from build123d import *

# Parameters (mm, degrees)
SKETCH1_R           = 5.75
BOSS_EXTRUDE1_DEPTH = 1
SKETCH2_R           = 5
BOSS_EXTRUDE2_DEPTH = 3
SKETCH3_R           = 1.5
CUT_EXTRUDE1_DEPTH  = 10.06228448
SKETCH4_R           = 762
SKETCH4_R_2         = 4
CUT_EXTRUDE2_DEPTH  = 0.08
CUT_EXTRUDE3_START  = -0.08
SKETCH5_R           = 4
SKETCH5_R_2         = 2.5
CUT_EXTRUDE3_DEPTH  = 0.08
FILLET1_R           = 0.31


with BuildPart() as part:
    # Sketch1 → Boss-Extrude1 (new body)
    with BuildSketch(Plane(origin=(0, 0, 0), x_dir=(1, 0, 0), z_dir=(0, 1, 0))):
        with Locations(Location((0, 0, 0), (0, 0, 270))):
            Circle(SKETCH1_R)
    extrude(amount=BOSS_EXTRUDE1_DEPTH)

    # Sketch2 → Boss-Extrude2 (add)
    with BuildSketch(Plane(origin=(0, 1, 0), x_dir=(1, 0, 0), z_dir=(0, 1, 0))):
        with Locations(Location((0, 0, 0), (0, 0, 270))):
            Circle(SKETCH2_R)
    extrude(amount=BOSS_EXTRUDE2_DEPTH)

    # Sketch3 → Cut-Extrude1 (cut, through all)
    with BuildSketch(Plane(origin=(0, 4, 0), x_dir=(1, 0, 0), z_dir=(0, 1, 0))):
        with Locations(Location((0, 0, 0), (0, 0, 270))):
            Circle(SKETCH3_R)
    extrude(amount=-CUT_EXTRUDE1_DEPTH, mode=Mode.SUBTRACT)

    # Sketch4 → Cut-Extrude2 (cut)
    with BuildSketch(Plane.XZ):
        Circle(SKETCH4_R)
        with Locations(Location((0, 0, 0), (0, 0, 270))):
            Circle(SKETCH4_R_2, mode=Mode.SUBTRACT)
    extrude(amount=-CUT_EXTRUDE2_DEPTH, mode=Mode.SUBTRACT)

    # Sketch5 → Cut-Extrude3 (cut)
    with BuildSketch(Plane(origin=(0, 4, 0), x_dir=(1, 0, 0), z_dir=(0, 1, 0)).offset(CUT_EXTRUDE3_START)):
        with Locations(Location((0, 0, 0), (0, 0, 90))):
            Circle(SKETCH5_R)
        with Locations(Location((0, 0, 0), (0, 0, 270))):
            Circle(SKETCH5_R_2, mode=Mode.SUBTRACT)
    extrude(amount=CUT_EXTRUDE3_DEPTH, mode=Mode.SUBTRACT)

    # Fillet1
    fillet1_edges = [part.edges().sort_by_distance(p)[0] for p in [
        (0, 0, -1.5),
        (0, 4, -1.5),
        (0, 4, -5),
    ]]
    fillet(fillet1_edges, radius=FILLET1_R)


solid = part.part
Build history of the part. All positions in model axes, mm. A direction names the side the tool comes from. Coordinates: 2 decimals unless noted, no trailing zeros. Order: outer loops, then holes, each group sorted by start corner. A loop starts at its lowest first (then second) coordinate and runs counter-clockwise, first axis right, second up. Notation, with made-up numbers: (-6.5, -9) -> (5.5, -9) arc R31 cw to (5.5, 24) -> close; hole circle Ø2 at (34, 61). An arc over 180 degrees is marked (long way). One line per item, written item: value.
(1) Probe line 1 (X direction, y = 1.9, z = 0); line 2 (X direction, y = 1.05, z = -1.25); line 3 (Y direction, x = -1, z = 5). List the from-to ranges inside material, lowest first. Write a range as [from, to].
Checked values:
line 1: [-5, -1.5], [1.5, 5]
line 2: [-4.84, -0.83], [0.83, 4.84]
line 3: [0.08, 1]
(2) Mould opens along X. For faces 1 (the cylindrical face through (0.45, 2.02, 1.43)), 2 (the flat face through (1, 4, 2)), 3 (the cylindrical face through (4.85, 0.53, 3.09)) say: pulls with the +X half, pulls with the -X half, needs draft (parallel to the pull), parting line crosses it, or undercut.
Checked values:
face 1: undercut
face 2: needs draft
face 3: parting line crosses it
(3) Tool access for faces 4 (the flat face through (2, 0.08, -4)), 5 (the flat face through (-1, 0, 2)), 6 (the flat face through (5, 1, -2)): list every direction of +Z, -Z, +X, -X, +Y, -Y with a clear straight run to the whole face (end or side of a thin tool).
Checked values:
face 4: -Y
face 5: +Z, -Z, +X, -X, -Y
face 6: +Y
(4) Slice it at D-D, the plane y = 0.5. List the corners of the cut face in (x, z), plus the area to 3 significant figures.
Checked values:
outline: circle Ø11.5 at (0, 0); hole circle Ø3 at (0, 0)
area: 96.8 mm2
(5) Drop a flat-ended pin along its axis: pin 1 Ø1.5 at (x, y) = (-1.5, 2.5) entering from -Z. Give the stop position or say it passes through.
Checked values:
pin 1: z = -4.94
(6) Slice it at C-C, the plane y = 2.5. List the corners of the cut face in (x, z), plus the area to 3 significant figures.
Checked values:
outline: circle Ø10 at (0, 0); hole circle Ø3 at (0, 0)
area: 71.5 mm2
